Here's how the part is built. I have some questions about the finished solid (model axes, mm). A direction names the side the tool comes from. Give positions to 0.01 mm unless a question says otherwise; leave off trailing zeros. Loops run counter-clockwise (first coordinate to the right, second up) from the corner with the lowest first, then second, coordinate; pieces in that order, holes last. Notation, with made-up numbers: M 22.25,-8 L 27.25,-8 A9 ccw 27.25,9 Z; hole C -29,37 d5. An arc over 180 degrees is marked long. Write item = value, one per line. Start each with the question number.
```python
from build123d import *

# Parameters (mm, degrees)
SKETCH1_W           = 177.8
SKETCH1_H           = 101.6
BOSS_EXTRUDE1_DEPTH = 6.35
BOSS_EXTRUDE2_DEPTH = 177.8
SKETCH3_W           = 57.658
SKETCH3_H           = 101.6
SKETCH3_W_2         = 4.2545
CUT_EXTRUDE1_DEPTH  = 127.448072965
FILLET1_R           = 43.18
FILLET2_R           = 12.7
SKETCH5_R           = 1
SKETCH5_W           = 13.335
SKETCH5_H           = 23.241
CUT_EXTRUDE2_DEPTH  = 177.112534328
CUT_EXTRUDE3_START  = 118.491
SKETCH5_2_R         = 1
SKETCH5_2_W         = 13.335
SKETCH5_2_H         = 23.241
CUT_EXTRUDE3_DEPTH  = 58.621534328
FILLET4_R           = 2.54


with BuildPart() as part:
    # Sketch1 → Boss-Extrude1 (new body)
    with BuildSketch(Plane(origin=(0, 0, 0), x_dir=(1, 0, 0), z_dir=(0, 1, 0))):
        Rectangle(SKETCH1_W, SKETCH1_H)
    extrude(amount=BOSS_EXTRUDE1_DEPTH)

    # Sketch2 → Boss-Extrude2 (add)
    with BuildSketch(Plane.ZY.offset(88.9)):
        with BuildLine():
            Line((0, 69.088), (0, 6.35))
            Line((0, 6.35), (10.287, 6.35))
            Line((10.287, 6.35), (10.287, 76.2))
            ThreePointArc((10.287, 76.2), (10.043157025, 78.426514309), (9.323188205, 80.547474059))
            Line((9.323188205, 80.547474059), (6.445660981, 79.205661077))
            ThreePointArc((6.445660981, 79.205661077), (5.998199963, 72.378725185), (0, 69.088))
        make_face()
        with BuildLine():
            Line((-10.287, 76.2), (-10.287, 6.35))
            Line((-10.287, 6.35), (0, 6.35))
            Line((0, 6.35), (0, 69.088))
            ThreePointArc((0, 69.088), (-5.998199963, 72.378725185), (-6.445660981, 79.205661077))
            Line((-6.445660981, 79.205661077), (-9.323188205, 80.547474059))
            ThreePointArc((-9.323188205, 80.547474059), (-10.043157025, 78.426514309), (-10.287, 76.2))
        make_face()
    extrude(amount=-BOSS_EXTRUDE2_DEPTH)

    # Sketch3 → Cut-Extrude1 (cut, through all)
    with BuildSketch(Plane(origin=(0, 6.35, 0), x_dir=(1, 0, 0), z_dir=(0, 1, 0))):
        with Locations((-30.4165, 0)):
            Rectangle(SKETCH3_W, SKETCH3_H)
        with Locations((30.4165, 0)):
            Rectangle(SKETCH3_W, SKETCH3_H)
        with Locations((86.77275, 0)):
            Rectangle(SKETCH3_W_2, SKETCH3_H)
        with Locations((-86.77275, 0)):
            Rectangle(SKETCH3_W_2, SKETCH3_H)
    extrude(amount=CUT_EXTRUDE1_DEPTH, mode=Mode.SUBTRACT)

    # Fillet1
    fillet1_edges = [part.edges().sort_by_distance(p)[0] for p in [
        (1.5875, 6.35, 0),
        (-1.5875, 6.35, 0),
    ]]
    fillet(fillet1_edges, radius=FILLET1_R)

    # Fillet2
    fillet2_edges = [part.edges().sort_by_distance(p)[0] for p in [
        (59.2455, 6.35, 0),
        (-59.2455, 6.35, 0),
    ]]
    fillet(fillet2_edges, radius=FILLET2_R)

    # Sketch5 → Cut-Extrude2 (cut, through all)
    with BuildSketch(Plane.ZY.offset(-59.2455)):
        with Locations((0, 54.7)):
            Circle(SKETCH5_R)
        with Locations((0, 27.014)):
            Circle(SKETCH5_R)
        with Locations((0, 40.9615)):
            Rectangle(SKETCH5_W, SKETCH5_H)
    extrude(amount=-CUT_EXTRUDE2_DEPTH, mode=Mode.SUBTRACT)

    # Sketch5<2> → Cut-Extrude3 (cut, through all)
    with BuildSketch(Plane.ZY.offset(-59.2455).offset(CUT_EXTRUDE3_START)):
        with Locations((0, 54.7)):
            Circle(SKETCH5_2_R)
        with Locations((0, 27.014)):
            Circle(SKETCH5_2_R)
        with Locations((0, 40.9615)):
            Rectangle(SKETCH5_2_W, SKETCH5_2_H)
    extrude(amount=CUT_EXTRUDE3_DEPTH, mode=Mode.SUBTRACT)

    # Fillet4
    fillet4_edges = [part.edges().sort_by_distance(p)[0] for p in [
        (71.9455, 79.205661077, -6.445660981),
        (0, 79.205661077, -6.445660981),
        (-71.9455, 79.205661077, -6.445660981),
        (71.9455, 79.205661077, 6.445660981),
        (0, 79.205661077, 6.445660981),
        (-71.9455, 79.205661077, 6.445660981),
    ]]
    fillet(fillet4_edges, radius=FILLET4_R)


solid = part.part
```
Q1. On a 3-axis mill with a long thin cutter (end or side, diameter ignored), from which of +Z, -Z, +X, -X, +Y, -Y can I reach the whole of each face in a straight line? I mean faces 1 (the flat face through (-84.646, 43, -7)), 2 (the cylindrical face through (-72.123, 78.457, -10.036)), 3 (the flat face through (59.246, 49, -7)), 4 (the flat face through (72, 52.582, 0)), 5 (the flat face through (-70, 41, 10.287)). Say none if no direction works.
Q2. We'd pull the mould along Z, two halves only. Please class faces 6 (the flat face through (0, 21, -10.287)), 7 (the cylindrical face through (14.572, 18.663, -0.144)), 8 (the flat face through (-1, 3, 50.8)), 9 (the flat face through (-72, 52.582, 0)): pulls with the +Z half, pulls with the -Z half, needs draft (parallel to the pull), parting line crosses it, or undercut.
Q3. Will these pins go through, and if not, where does the flat tip stop? pin 1 (10.5 mm diameter, centred on y = 66.5, z = 1, fed in from -X); pin 2 (3 mm diameter, centred on y = 54.7, z = 0, fed in from +X); pin 3 (1.5 mm diameter, centred on x = 29.5, z = 36.5, fed in from +Y); pin 4 (1 mm diameter, centred on x = 4, y = 60, fed in from -Z).
Q4. If we section it at A-A, the plane y = 33.5: List the corners of the cut face in (x, z) for me.
Q5. If we section it at B-B, the plane x = 67: List the corners of the cut face in (y, z) for me.
Q6. If we section it at C-C, the plane z = -26: List the corners of the cut face in (x, y) for me.
Q7. If I drill on line 1 along Y through (x, z) = (-78, 0); line 2 along X through (y, z) = (65, 9); line 3 along Z through (x, y) = (-73.5, 54.7), over which ranges is the centre line in solid material (lowest first)?
Resolved:
q1.face_1 = +Z, -Z, -X, +Y
q1.face_2 = -Z, +X, -X, +Y
q1.face_3 = +Z, -Z, +Y
q1.face_4 = +X
q1.face_5 = +Z, +X, -X, +Y
q2.face_6 = pulls with the -Z half
q2.face_7 = needs draft
q2.face_8 = pulls with the +Z half
q2.face_9 = undercut
q3.pin_1 = -84.65
q3.pin_2 = 84.65
q3.pin_3 = 6.35
q3.pin_4 = through
q4.outline = M -84.65,-10.29 L -59.25,-10.29 L -59.25,-6.67 L -84.65,-6.67 Z; M -84.65,6.67 L -59.25,6.67 L -59.25,10.29 L -84.65,10.29 Z; M -4.67,-10.29 L 4.67,-10.29 L 4.67,10.29 L -4.67,10.29 Z; M 59.25,-10.29 L 84.65,-10.29 L 84.65,-6.67 L 59.25,-6.67 Z; M 59.25,6.67 L 84.65,6.67 L 84.65,10.29 L 59.25,10.29 Z
q5.outline = M 0,-50.8 L 6.35,-50.8 L 6.35,-10.29 L 76.2,-10.29 A10.29 ccw 80.55,-9.32 L 80.14,-8.44 A2.54 ccw 77.4,-7.01 A7.11 cw long 77.4,7.01 A2.54 ccw 80.14,8.44 L 80.55,9.32 A10.29 ccw 76.2,10.29 L 6.35,10.29 L 6.35,50.8 L 0,50.8 Z; hole C 27.01,0 d2; hole M 29.34,-6.67 L 52.58,-6.67 L 52.58,6.67 L 29.34,6.67 Z; hole C 54.7,0 d2
q6.outline = M -88.9,0 L 88.9,0 L 88.9,6.35 L -88.9,6.35 Z
q7.line_1 = 0 to 26.01, 28.01 to 29.34, 52.58 to 53.7, 55.7 to 69.09
q7.line_2 = -84.65 to -59.25, -1.59 to 1.59, 59.25 to 84.65
q7.line_3 = -10.29 to -1, 1 to 10.29
